Autodesk Inventor part; units mm, degrees
ref_plane "YZ Plane" through (0, 0, 0) normal (1, 0, 0) x (0, 1, 0)
ref_plane "XZ Plane" through (0, 0, 0) normal (0, 1, 0) x (-1, 0, 0)
ref_plane "XY Plane" through (0, 0, 0) normal (0, 0, 1) x (1, 0, 0)
sketch "Skizze1" plane through (0, 0, 0) normal (0, 0, 1) x (1, 0, 0)
  line L0 (-9.8, 0) -> (9.8, 0)
  line L1 (0, -9.8) -> (0, 9.8)
  circle A0 centre (0, 0) radius 7
  point P0 (0, 7)
  point P1 (-7, 0)
  point P2 (0, -7)
  point P3 (7, 0)
  dimension "d19" = 14
extrude "Extrusion1" add sketch "Skizze1" along normal blind 2
sketch "Skizze2" plane through (0, 0, 0) normal (0, 0, -1) x (-1, 0, 0)
  circle A0 centre (0, 0) radius 7.5
  dimension "d7" = 15
extrude "Extrusion2" add sketch "Skizze2" along normal blind 5
chamfer "Fase2" distance 0.5 angle 45 2 edges at (7.5, 0, 0) (7.5, 0, -5)
sketch "Skizze4" plane through (0, 0, 2) normal (0, 0, 1) x (1, 0, 0)
  circle A0 centre (0, 0) radius 6.58
  dimension "d20" = 13.16
extrude "Extrusion4" add sketch "Skizze4" along normal blind 8
thread "Gewinde2"
chamfer "Fase4" distance 0.5 angle 45 1 edges at (-6.58, 0, 10)
sketch "Skizze5" plane through (0, 0, -5) normal (0, 0, -1) x (-1, 0, 0)
  circle A0 centre (0, 0) radius 4
  dimension "d28" = 8
extrude "Extrusion5" cut sketch "Skizze5" against normal blind 15
chamfer "Fase5" distance 0.5 angle 45 1 edges at (4, 0, -5)
properties part number "Schlauchsteckverbindung"
Source: CAD feature listing. Evaluate the final solid. Frame: model axes, mm. A direction names the side the tool comes from. Coordinates: 2 decimals unless noted, no trailing zeros. Order: outer loops, then holes, each group sorted by start corner. A loop starts at its lowest first (then second) coordinate and runs counter-clockwise, first axis right, second up. Notation, with made-up numbers: M 62,89.25 L 73,89.25 A30 cw 73,123.25 Z; hole C 4.5,75.25 d10. An arc over 180 degrees is marked long. Write each question's results on one line, items separated by ' | '. Start each with the question number.
Item 1: Draft query along Y for faces 3 (the face through (0.867, -3.905, 2.649)), 4 (the face through (-5, 0, -5)), 5 (the face through (6.466, 2.681, 0.986)). Return one class per face: pulls with the +Y half, pulls with the -Y half, needs draft (parallel to the pull), parting line crosses it, or undercut.
Item 2: Set-up query: faces 1 (the face through (4, -1.3, 10)), 2 (the face through (-1.426, 6.424, 5.698)). Return all of +Z, -Z, +X, -X, +Y, -Y with unobstructed straight access to the full face (end or side cutting, diameter ignored); none if empty.
Item 3: Line query: probe 1 along Y at (x, z) = (0, 6); probe 2 along Y at (x, z) = (-6, -3.75); probe 3 along Y at (x, z) = (3.5, -4). Output: solid intervals per line, ascending.
Item 4: First-contact query: pin 1 Ø4 at (x, z) = (0.5, 8) entering from -Y; pin 2 Ø7 at (x, y) = (0, 0) entering from -Z; pin 3 Ø8 at (y, z) = (1, 3.5) entering from +X. Flat tips, straight axial feed; report the tip coordinate or a pass-through.
Item 5: Cut plane D-D (z = -3.75). Return loops of the section in (x, y).
Item 6: Cut plane C-C (z = 8.5). Return loops of the section in (x, y).
Checked values:
1) face 3: undercut | face 4: needs draft | face 5: parting line crosses it
2) face 1: +Z, +X, -X, +Y, -Y | face 2: +Z
3) probe 1: y = -6.58 to -4, 4 to 6.58 | probe 2: y = -4.5 to 4.5 | probe 3: y = -6.63 to -1.94, 1.94 to 6.63
4) pin 1: stops at y = -6.58 | pin 2: passes through | pin 3: stops at x = 7.46
5) outline: C 0,0 d15; hole C 0,0 d8
6) outline: C 0,0 d13.16; hole C 0,0 d8
